```python
from build123d import *

# Parameters (mm, degrees)
BOSS_EXTRUDE1_DEPTH                                 = 5
SKETCH2_R                                           = 2.5
CUT_EXTRUDE1_DEPTH                                  = 6
CSK_FOR_M3_COUNTERSUNK_FLAT_HEAD_SCREW1_D           = 3.4
CSK_FOR_M3_COUNTERSUNK_FLAT_HEAD_SCREW1_DEPTH       = 5
CSK_FOR_M3_COUNTERSUNK_FLAT_HEAD_SCREW1_CSINK_D     = 6.3
CSK_FOR_M3_COUNTERSUNK_FLAT_HEAD_SCREW1_CSINK_ANGLE = 90


with BuildPart() as part:
    # Sketch1 → Boss-Extrude1 (new body)
    with BuildSketch(Plane.XY):
        with BuildLine():
            Line((4, 10), (4, 28))
            ThreePointArc((4, 28), (0, 32), (-4, 28))
            Line((-4, 28), (-4, 10))
            Line((-4, 10), (-15, 10))
            Line((-15, 10), (-15, 0))
            Line((-15, 0), (15, 0))
            Line((15, 0), (15, 10))
            Line((15, 10), (4, 10))
        make_face()
    extrude(amount=BOSS_EXTRUDE1_DEPTH)

    # Sketch2 → Cut-Extrude1 (cut, through all)
    with BuildSketch(Plane.XY.offset(5)):
        with Locations((0, 28)):
            Circle(SKETCH2_R)
    extrude(amount=-CUT_EXTRUDE1_DEPTH, mode=Mode.SUBTRACT)

    # CSK for M3 Countersunk Flat Head Screw1
    with Locations(Plane(origin=(0, 0, 0), x_dir=(-1, 0, 0), z_dir=(0, 0, -1))):
        with Locations((0, 5), (11, 5), (-11, 5)):
            CounterSinkHole(CSK_FOR_M3_COUNTERSUNK_FLAT_HEAD_SCREW1_D / 2, CSK_FOR_M3_COUNTERSUNK_FLAT_HEAD_SCREW1_CSINK_D / 2, depth=CSK_FOR_M3_COUNTERSUNK_FLAT_HEAD_SCREW1_DEPTH, counter_sink_angle=CSK_FOR_M3_COUNTERSUNK_FLAT_HEAD_SCREW1_CSINK_ANGLE)


solid = part.part
```
Here's how the part is built. I have some questions about the finished solid (model axes, mm). A direction names the side the tool comes from. Round coordinates to 2 decimals unless told otherwise and drop trailing zeros. Loops run counter-clockwise (first coordinate to the right, second up) from the corner with the lowest first, then second, coordinate; pieces in that order, holes last.
1. Suppose I cut it at D-D, the plane z = 3.45. Please give me the cut outline in (x, y).
Answers:
outline: (-15, 0) - (15, 0) - (15, 10) - (4, 10) - (4, 28) arc R4 ccw to (-4, 28) - (-4, 10) - (-15, 10) - close; hole circle Ø3.4 at (-11, 5); hole circle Ø5 at (0, 28); hole circle Ø3.4 at (0, 5); hole circle Ø3.4 at (11, 5)
2. Thinking about a two-plate mould opening in X: for faces 1 (the face through (-15, 5, 2)), 2 (the face through (-9, 10, 2)), 3 (the face through (11.8, 3.5, 3.2)), which applies, released by +X, released by -X, zero draft, split by the parting line, or undercut?
Answers:
face 1: released by -X
face 2: zero draft
face 3: undercut
3. If I drill on probe 1 along X at (y, z) = (5, 4.15); probe 2 along Y at (x, z) = (0, 1.65); probe 3 along X at (y, z) = (4.5, 1.1), over which ranges is the centre line in solid material (lowest first)?
Answers:
probe 1: x = -15 to -12.7, -9.3 to -1.7, 1.7 to 9.3, 12.7 to 15
probe 2: y = 0 to 3.3, 6.7 to 25.5, 30.5 to 32
probe 3: x = -15 to -12.99, -9.01 to -1.99, 1.99 to 9.01, 12.99 to 15
4. Suppose I cut it at A-A, the plane y = 5. Please give me the cut outline in (x, z), and give its area (3 significant figures).
Answers:
outline: (-15, 0) - (-14.15, 0) - (-12.7, 1.45) - (-12.7, 5) - (-15, 5) - close; (-9.3, 1.45) - (-7.85, 0) - (-3.15, 0) - (-1.7, 1.45) - (-1.7, 5) - (-9.3, 5) - close; (1.7, 1.45) - (3.15, 0) - (7.85, 0) - (9.3, 1.45) - (9.3, 5) - (1.7, 5) - close; (12.7, 1.45) - (14.15, 0) - (15, 0) - (15, 5) - (12.7, 5) - close
area: 92.7 mm2
5. For faces 4 (the face through (10, 10, 2)), 5 (the face through (-4, 19, 2)), 6 (the face through (15, 5, 2)), which set-ups out of +Z, -Z, +X, -X, +Y, -Y let a thin tool reach every point of the face, with its end or its side?
Answers:
face 4: +Z, -Z, +X, +Y
face 5: +Z, -Z, -X, +Y
face 6: +Z, -Z, +X, +Y, -Y
6. Will these pins go through, and if not, where does the flat tip stop? pin 1 (1.5 mm diameter, centred on y = 19.5, z = 2, fed in from +X); pin 2 (1.5 mm diameter, centred on x = -7.5, z = 2, fed in from +Y).
Answers:
pin 1: stops at x = 4
pin 2: stops at y = 10
7. Suppose I cut it at C-C, the plane x = -11. Please give me the cut outline in (y, z).
Answers:
outline: (0, 0) - (1.85, 0) - (3.3, 1.45) - (3.3, 5) - (0, 5) - close; (6.7, 1.45) - (8.15, 0) - (10, 0) - (10, 5) - (6.7, 5) - close
8. Suppose I cut it at B-B, the plane z = 0.55. Please give me the cut outline in (x, y).
Answers:
outline: (-15, 0) - (15, 0) - (15, 10) - (4, 10) - (4, 28) arc R4 ccw to (-4, 28) - (-4, 10) - (-15, 10) - close; hole circle Ø5.2 at (-11, 5); hole circle Ø5.2 at (0, 5); hole circle Ø5 at (0, 28); hole circle Ø5.2 at (11, 5)
